Work out the finished part from the listing and answer in its coordinate system (mm). Face numbers are marked on the shaded views. Coordinates: 2 decimals unless noted, no trailing zeros. Loops run counter-clockwise (first coordinate to the right, second up) from the corner with the lowest first, then second, coordinate; pieces in that order, holes last.
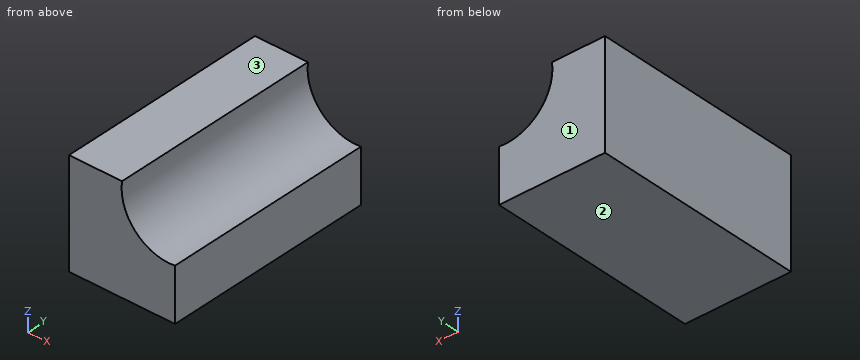
```python
from build123d import *

# Parameters (mm, degrees)
F1_DEPTH = 50.8


with BuildPart() as f1:
    # F0 (on Front) → F1 (new body)
    with BuildSketch(Plane.XZ):
        with BuildLine():
            Line((-25.4, 0), (0, 0))
            Line((0, 0), (0, 12.7))
            ThreePointArc((0, 12.7), (-9.495563, 15.904437), (-12.7, 25.4))
            Line((-12.7, 25.4), (-25.4, 25.4))
            Line((-25.4, 25.4), (-25.4, 0))
        make_face()
    extrude(amount=F1_DEPTH)


solid = f1.part
```
1. A cutting plane is placed at A-A, the plane y = -36. Give the vertices of the cut face in (x, z), then the cut area to 3 significant figures.
2. Determine the mould class of the marked faces 1, 2 and 3 for opening direction Z: released by +Z, released by -Z, zero draft, split by the parting line, or undercut.
3. A cutting plane is placed at C-C, the plane z = 14.25. Give the vertices of the cut face in (x, y).
4. A cutting plane is placed at B-B, the plane x = -2.75. Give the vertices of the cut face in (y, z), then the cut area to 3 significant figures.
5. Straight lines are drawn through the part: probe 1 along X at (y, z) = (-35, 17.25); probe 2 along Z at (x, y) = (-8.5, -17.5); probe 3 along Z at (x, y) = (-1.5, -42.5). For each, find the intervals that lie inside material, in ascending order.
Answers below:
1. outline: (-25.4, 0) - (0, 0) - (0, 12.7) arc R11.29 cw to (-12.7, 25.4) - (-25.4, 25.4) - close
1. area: 509 mm2
2. face 1: zero draft
2. face 2: released by -Z
2. face 3: released by +Z
3. outline: (-25.4, -50.8) - (-7.39, -50.8) - (-7.39, 0) - (-25.4, 0) - close
4. outline: (-50.8, 0) - (0, 0) - (0, 12.67) - (-50.8, 12.67) - close
4. area: 643 mm2
5. probe 1: x = -25.4 to -10.64
5. probe 2: z = 0 to 15.02
5. probe 3: z = 0 to 12.6
